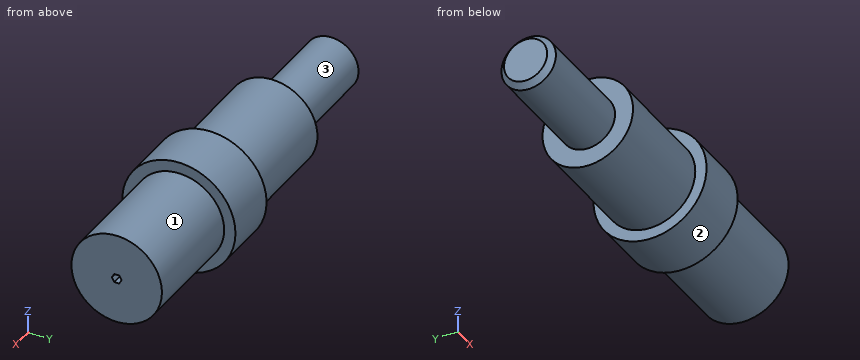
from build123d import *

# Parameters (mm, degrees)
F0_R      = 20
F1_DEPTH  = 20
F2_R      = 16
F3_DEPTH  = 40
F4_R      = 9.625258
F5_DEPTH  = 40
F6_SIZE   = 2
F7_R      = 16
F8_DEPTH  = 40
F10_DEPTH = 10.2


with BuildPart() as f1:
    # F0 (on Right) → F1 (new body)
    with BuildSketch(Plane.YZ):
        Circle(F0_R)
    extrude(amount=-F1_DEPTH)

    # F2 (on face) → F3 (join)
    with BuildSketch(Plane(origin=(-20, 0, 0), x_dir=(0, -1, 0), z_dir=(-1, 0, 0))):
        Circle(F2_R)
    extrude(amount=F3_DEPTH)

    # F4 (on face) → F5 (join)
    with BuildSketch(Plane(origin=(-60, 0, 0), x_dir=(0, -1, 0), z_dir=(-1, 0, 0))):
        Circle(F4_R)
    extrude(amount=F5_DEPTH)

    # F6
    f6_edges = [f1.edges().sort_by_distance(p)[0] for p in [
        (-100, 9.625258, 0),
    ]]
    chamfer(f6_edges, length=F6_SIZE)

    # F7 (on face) → F8 (join)
    with BuildSketch(Plane.YZ):
        Circle(F7_R)
    extrude(amount=F8_DEPTH)

    # F9 (on face) → F10 (cut)
    with BuildSketch(Plane.YZ.offset(40)):
        Polygon((-0.866025, -1.5), (0.866025, -1.5), (1.732051, 0), (0.866025, 1.5), (-0.866025, 1.5), (-1.732051, 0), align=None)
    extrude(amount=-F10_DEPTH, mode=Mode.SUBTRACT)


solid = f1.part
Check sheet for the modelled part. Datum: model origin and axes. Units: mm. Face numbers are marked on the shaded views. A direction names the side the tool comes from. Give positions to 0.01 mm unless a question says otherwise; leave off trailing zeros. Loops run counter-clockwise (first coordinate to the right, second up) from the corner with the lowest first, then second, coordinate; pieces in that order, holes last. Notation, with made-up numbers: M 33,32 L 40,32 A29 cw 40,54 Z; hole C -14,26 d1. An arc over 180 degrees is marked long. Use a Markdown table: item, result. Add a question column.
Q1. Sectioned sample at A-A, the plane z = 13.5. Record the cut outline in (x, y), then the cut area to 3 significant figures.
Q2. Go/stop test with flat-tipped pins: pin 1 (4 mm diameter, centred on x = -84, y = -7.5, fed in from -Z); pin 2 (0.9 mm diameter, centred on x = 35, y = 0, fed in from +Z); pin 3 (10 mm diameter, centred on x = -67.5, y = -8.5, fed in from -Z). Record where each tip stops, or that it passes through.
Q3. Sectioned sample at B-B, the plane x = 7.5. Record the cut outline in (y, z).
Q4. Tool access check on the marked faces 1, 2 and 3. Record the directions out of +Z, -Z, +X, -X, +Y, -Y that give a thin tool (end or side, any length) a straight path to the whole face; none if there is none.
Q5. Scan lines: line 1 along X through (y, z) = (4, -17.5); line 2 along X through (y, z) = (0.5, 0); line 3 along Z through (x, y) = (31.5, -11). Record each from-to range of solid material in increasing order. Write a range as [from, to].
Q6. Sectioned sample at C-C, the plane y = -11. Record the cut outline in (x, z).
Verdict:
| question | item | result |
|---|---|---|
| 1 | outline | M -60,-8.59 L -20,-8.59 L -20,-14.76 L 0,-14.76 L 0,-8.59 L 40,-8.59 L 40,8.59 L 0,8.59 L 0,14.76 L -20,14.76 L -20,8.59 L -60,8.59 Z |
| 1 | area | 1,960 mm^2 |
| 2 | pin 1 | z = -7.9 |
| 2 | pin 2 | z = 16 |
| 2 | pin 3 | z = -8.97 |
| 3 | outline | C 0,0 d32 |
| 4 | face 1 | +X |
| 4 | face 2 | +X, -X |
| 4 | face 3 | -X |
| 5 | line 1 | [-20, 0] |
| 5 | line 2 | [-100, 29.8] |
| 5 | line 3 | [-11.62, 11.62] |
| 6 | outline | M -60,-11.62 L -20,-11.62 L -20,-16.7 L 0,-16.7 L 0,-11.62 L 40,-11.62 L 40,11.62 L 0,11.62 L 0,16.7 L -20,16.7 L -20,11.62 L -60,11.62 Z |
